Design review of the part built by this model. Coordinates are the model's own, in mm. Give positions to 0.01 mm unless a question says otherwise; leave off trailing zeros. Write each loop counter-clockwise with the first axis right and the second up, starting at its lowest first coordinate (ties: lowest second). Pieces come first, ordered by that corner, then holes. Notation, with made-up numbers: M 37,19 L 43,19 A23 ccw 43,36 Z; hole C -6,61 d1. An arc over 180 degrees is marked long. Use a Markdown table: item, result. Add a question column.
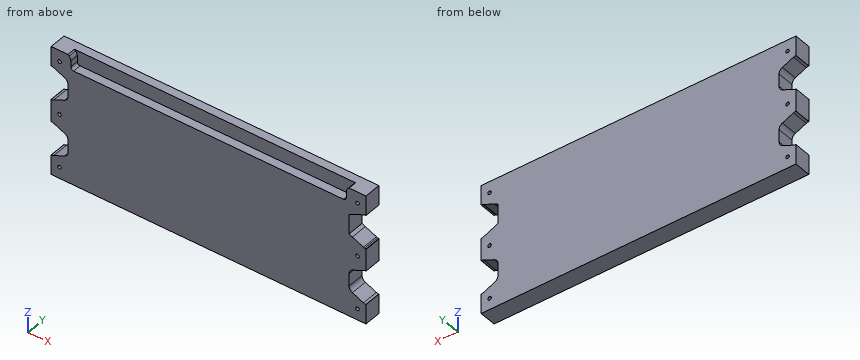
```python
from build123d import *

# Parameters (mm, degrees)
F0_R     = 1.984375
F1_DEPTH = 9.525
F2_DEPTH = 9.525
F3_SIZE  = 3.175
F4_R     = 6.35


# Not quite as in the source:
# - ends of sketch curves that miss each other by under 0.0002 mm in the source are joined


with BuildPart() as f1:
    # F0 (on Front) → F1 (new body)
    with BuildSketch(Plane.XZ):
        with BuildLine():
            ThreePointArc((106.6892375248, 39.5968594302), (108.9343015551, 40.5267953999), (109.8642375248, 42.7718594302))
            Line((109.8642375248, 42.7718594302), (109.8642375248, 55.4718594302))
            Line((109.8642375248, 55.4718594302), (-201.2857624752, 55.4718594302))
            Line((-201.2857624752, 55.4718594302), (-201.2857624752, 42.7718594302))
            ThreePointArc((-201.2857624752, 42.7718594302), (-200.3558265055, 40.5267953999), (-198.1107624752, 39.5968594302))
            Line((-198.1107624752, 39.5968594302), (106.6892375248, 39.5968594302))
        make_face()
        with BuildLine():
            Line((109.8642375248, 55.4718594302), (109.8642375248, 42.7718594302))
            ThreePointArc((109.8642375248, 42.7718594302), (108.9343015551, 40.5267953999), (106.6892375248, 39.5968594302))
            Line((106.6892375248, 39.5968594302), (-198.1107624752, 39.5968594302))
            ThreePointArc((-198.1107624752, 39.5968594302), (-200.3558265055, 40.5267953999), (-201.2857624752, 42.7718594302))
            Line((-201.2857624752, 42.7718594302), (-201.2857624752, 55.4718594302))
            Line((-201.2857624752, 55.4718594302), (-223.5107624752, 55.4718594302))
            Line((-223.5107624752, 55.4718594302), (-223.5107624752, 33.2468594302))
            Line((-223.5107624752, 33.2468594302), (-223.2986885503, 33.2468594302))
            ThreePointArc((-223.2986885503, 33.2468594302), (-221.9543922864, 33.1029344825), (-220.6710339026, 32.6776838569))
            Line((-220.6710339026, 32.6776838569), (-208.1831078275, 27.0013383101))
            ThreePointArc((-208.1831078275, 27.0013383101), (-205.471843717, 24.6583106333), (-204.4607624752, 21.2205138834))
            Line((-204.4607624752, 21.2205138834), (-204.4607624752, 7.1731958926))
            ThreePointArc((-204.4607624752, 7.1731958926), (-205.4718446589, 3.7353976799), (-208.1831109951, 1.392370026))
            Line((-208.1831109951, 1.392370026), (-220.6710352489, -4.2839664363))
            ThreePointArc((-220.6710352489, -4.2839664363), (-221.9543921654, -4.7092159904), (-223.298686729, -4.8531405698))
            Line((-223.298686729, -4.8531405698), (-223.5107370752, -4.8531405698))
            Line((-223.5107370752, -4.8531405698), (-223.5107624752, -30.2531405698))
            Line((-223.5107624752, -30.2531405698), (-223.298686729, -30.2531405698))
            ThreePointArc((-223.298686729, -30.2531405698), (-221.9543921654, -30.3970651492), (-220.6710352489, -30.8223147033))
            Line((-220.6710352489, -30.8223147033), (-208.1831109951, -36.4986511657))
            ThreePointArc((-208.1831109951, -36.4986511657), (-205.4718446589, -38.8416788196), (-204.4607624752, -42.2794770322))
            Line((-204.4607624752, -42.2794770322), (-204.4607624752, -56.326795023))
            ThreePointArc((-204.4607624752, -56.326795023), (-205.471843717, -59.7645917729), (-208.1831078275, -62.1076194497))
            Line((-208.1831078275, -62.1076194497), (-220.6710339026, -67.7839649965))
            ThreePointArc((-220.6710339026, -67.7839649965), (-221.9543922864, -68.2092156221), (-223.2986885503, -68.3531405698))
            Line((-223.2986885503, -68.3531405698), (-223.5107370752, -68.3531405698))
            Line((-223.5107370752, -68.3531405698), (-223.5107624752, -90.5781405698))
            Line((-223.5107624752, -90.5781405698), (132.0892375248, -90.5781405698))
            Line((132.0892375248, -90.5781405698), (132.0892375248, -68.3531405698))
            Line((132.0892375248, -68.3531405698), (131.8771635999, -68.3531405698))
            ThreePointArc((131.8771635999, -68.3531405698), (130.532867336, -68.2092156221), (129.2495089522, -67.7839649965))
            Line((129.2495089522, -67.7839649965), (116.7615828771, -62.1076194497))
            ThreePointArc((116.7615828771, -62.1076194497), (114.0503187666, -59.7645917729), (113.0392375248, -56.326795023))
            Line((113.0392375248, -56.326795023), (113.0392375248, -42.2794770322))
            ThreePointArc((113.0392375248, -42.2794770322), (114.0503197085, -38.8416788196), (116.7615860447, -36.4986511657))
            Line((116.7615860447, -36.4986511657), (129.2495102985, -30.8223147033))
            ThreePointArc((129.2495102985, -30.8223147033), (130.5328672149, -30.3970651492), (131.8771617786, -30.2531405698))
            Line((131.8771617786, -30.2531405698), (132.0892121248, -30.2531405698))
            Line((132.0892121248, -30.2531405698), (132.0892375248, -5.5747531892))
            Line((132.0892375248, -5.5747531892), (130.5016917914, -4.8531405698))
            Line((130.5016917914, -4.8531405698), (129.2495102985, -4.2839664363))
            Line((129.2495102985, -4.2839664363), (116.7615860447, 1.392370026))
            Line((116.7615860447, 1.392370026), (113.0392375248, 3.0843487889))
            Line((113.0392375248, 3.0843487889), (113.0392375248, 7.1731958926))
            Line((113.0392375248, 7.1731958926), (113.0392375248, 21.2205138834))
            Line((113.0392375248, 21.2205138834), (113.0392375248, 25.3093700715))
            Line((113.0392375248, 25.3093700715), (116.7615794549, 27.001345839))
            Line((116.7615794549, 27.001345839), (129.2495086403, 32.677684543))
            Line((129.2495086403, 32.677684543), (130.5016917914, 33.2468594302))
            Line((130.5016917914, 33.2468594302), (132.0892375248, 33.9684720496))
            Line((132.0892375248, 33.9684720496), (132.0892375248, 55.4718594302))
            Line((132.0892375248, 55.4718594302), (109.8642375248, 55.4718594302))
        make_face()
        with Locations((-213.9857624752, -77.8781405698)):
            Circle(F0_R, mode=Mode.SUBTRACT)
        with Locations((122.5642375248, -77.8781405698)):
            Circle(F0_R, mode=Mode.SUBTRACT)
        with Locations((-213.9857624752, -17.5531402737)):
            Circle(F0_R, mode=Mode.SUBTRACT)
        with Locations((-213.9857624752, 42.7718594302)):
            Circle(F0_R, mode=Mode.SUBTRACT)
        with Locations((122.5642375248, -17.5531402737)):
            Circle(F0_R, mode=Mode.SUBTRACT)
        with Locations((122.5642375248, 42.7718594302)):
            Circle(F0_R, mode=Mode.SUBTRACT)
        Polygon((132.0892375248, 33.2468594302), (132.0892375248, 33.9684720496), (130.5016917914, 33.2468594302), (131.8771635999, 33.2468594302), align=None)
        Polygon((132.0892375248, -5.5747531892), (132.0892375248, -4.8531405698), (131.8771617786, -4.8531405698), (130.5016917914, -4.8531405698), align=None)
    extrude(amount=-F1_DEPTH)

    # F0 (on Front) → F2 (join)
    with BuildSketch(Plane.XZ):
        with BuildLine():
            Line((109.8642375248, 55.4718594302), (109.8642375248, 42.7718594302))
            ThreePointArc((109.8642375248, 42.7718594302), (108.9343015551, 40.5267953999), (106.6892375248, 39.5968594302))
            Line((106.6892375248, 39.5968594302), (-198.1107624752, 39.5968594302))
            ThreePointArc((-198.1107624752, 39.5968594302), (-200.3558265055, 40.5267953999), (-201.2857624752, 42.7718594302))
            Line((-201.2857624752, 42.7718594302), (-201.2857624752, 55.4718594302))
            Line((-201.2857624752, 55.4718594302), (-223.5107624752, 55.4718594302))
            Line((-223.5107624752, 55.4718594302), (-223.5107624752, 33.2468594302))
            Line((-223.5107624752, 33.2468594302), (-223.2986885503, 33.2468594302))
            ThreePointArc((-223.2986885503, 33.2468594302), (-221.9543922864, 33.1029344825), (-220.6710339026, 32.6776838569))
            Line((-220.6710339026, 32.6776838569), (-208.1831078275, 27.0013383101))
            ThreePointArc((-208.1831078275, 27.0013383101), (-205.471843717, 24.6583106333), (-204.4607624752, 21.2205138834))
            Line((-204.4607624752, 21.2205138834), (-204.4607624752, 7.1731958926))
            ThreePointArc((-204.4607624752, 7.1731958926), (-205.4718446589, 3.7353976799), (-208.1831109951, 1.392370026))
            Line((-208.1831109951, 1.392370026), (-220.6710352489, -4.2839664363))
            ThreePointArc((-220.6710352489, -4.2839664363), (-221.9543921654, -4.7092159904), (-223.298686729, -4.8531405698))
            Line((-223.298686729, -4.8531405698), (-223.5107370752, -4.8531405698))
            Line((-223.5107370752, -4.8531405698), (-223.5107624752, -30.2531405698))
            Line((-223.5107624752, -30.2531405698), (-223.298686729, -30.2531405698))
            ThreePointArc((-223.298686729, -30.2531405698), (-221.9543921654, -30.3970651492), (-220.6710352489, -30.8223147033))
            Line((-220.6710352489, -30.8223147033), (-208.1831109951, -36.4986511657))
            ThreePointArc((-208.1831109951, -36.4986511657), (-205.4718446589, -38.8416788196), (-204.4607624752, -42.2794770322))
            Line((-204.4607624752, -42.2794770322), (-204.4607624752, -56.326795023))
            ThreePointArc((-204.4607624752, -56.326795023), (-205.471843717, -59.7645917729), (-208.1831078275, -62.1076194497))
            Line((-208.1831078275, -62.1076194497), (-220.6710339026, -67.7839649965))
            ThreePointArc((-220.6710339026, -67.7839649965), (-221.9543922864, -68.2092156221), (-223.2986885503, -68.3531405698))
            Line((-223.2986885503, -68.3531405698), (-223.5107370752, -68.3531405698))
            Line((-223.5107370752, -68.3531405698), (-223.5107624752, -90.5781405698))
            Line((-223.5107624752, -90.5781405698), (132.0892375248, -90.5781405698))
            Line((132.0892375248, -90.5781405698), (132.0892375248, -68.3531405698))
            Line((132.0892375248, -68.3531405698), (131.8771635999, -68.3531405698))
            ThreePointArc((131.8771635999, -68.3531405698), (130.532867336, -68.2092156221), (129.2495089522, -67.7839649965))
            Line((129.2495089522, -67.7839649965), (116.7615828771, -62.1076194497))
            ThreePointArc((116.7615828771, -62.1076194497), (114.0503187666, -59.7645917729), (113.0392375248, -56.326795023))
            Line((113.0392375248, -56.326795023), (113.0392375248, -42.2794770322))
            ThreePointArc((113.0392375248, -42.2794770322), (114.0503197085, -38.8416788196), (116.7615860447, -36.4986511657))
            Line((116.7615860447, -36.4986511657), (129.2495102985, -30.8223147033))
            ThreePointArc((129.2495102985, -30.8223147033), (130.5328672149, -30.3970651492), (131.8771617786, -30.2531405698))
            Line((131.8771617786, -30.2531405698), (132.0892121248, -30.2531405698))
            Line((132.0892121248, -30.2531405698), (132.0892375248, -5.5747531892))
            Line((132.0892375248, -5.5747531892), (130.5016917914, -4.8531405698))
            Line((130.5016917914, -4.8531405698), (129.2495102985, -4.2839664363))
            Line((129.2495102985, -4.2839664363), (116.7615860447, 1.392370026))
            Line((116.7615860447, 1.392370026), (113.0392375248, 3.0843487889))
            Line((113.0392375248, 3.0843487889), (113.0392375248, 7.1731958926))
            Line((113.0392375248, 7.1731958926), (113.0392375248, 21.2205138834))
            Line((113.0392375248, 21.2205138834), (113.0392375248, 25.3093700715))
            Line((113.0392375248, 25.3093700715), (116.7615794549, 27.001345839))
            Line((116.7615794549, 27.001345839), (129.2495086403, 32.677684543))
            Line((129.2495086403, 32.677684543), (130.5016917914, 33.2468594302))
            Line((130.5016917914, 33.2468594302), (132.0892375248, 33.9684720496))
            Line((132.0892375248, 33.9684720496), (132.0892375248, 55.4718594302))
            Line((132.0892375248, 55.4718594302), (109.8642375248, 55.4718594302))
        make_face()
        with Locations((-213.9857624752, -77.8781405698)):
            Circle(F0_R, mode=Mode.SUBTRACT)
        with Locations((122.5642375248, -77.8781405698)):
            Circle(F0_R, mode=Mode.SUBTRACT)
        with Locations((-213.9857624752, -17.5531402737)):
            Circle(F0_R, mode=Mode.SUBTRACT)
        with Locations((-213.9857624752, 42.7718594302)):
            Circle(F0_R, mode=Mode.SUBTRACT)
        with Locations((122.5642375248, -17.5531402737)):
            Circle(F0_R, mode=Mode.SUBTRACT)
        with Locations((122.5642375248, 42.7718594302)):
            Circle(F0_R, mode=Mode.SUBTRACT)
        Polygon((132.0892375248, 33.2468594302), (132.0892375248, 33.9684720496), (130.5016917914, 33.2468594302), (131.8771635999, 33.2468594302), align=None)
        Polygon((132.0892375248, -5.5747531892), (132.0892375248, -4.8531405698), (131.8771617786, -4.8531405698), (130.5016917914, -4.8531405698), align=None)
    extrude(amount=F2_DEPTH)

    # F3
    f3_edges = [f1.edges().sort_by_distance(p)[0] for p in [
        (-201.285762, -4.7625, 55.471859),
        (109.864238, -4.7625, 55.471859),
    ]]
    chamfer(f3_edges, length=F3_SIZE)

    # F4
    f4_edges = [f1.edges().sort_by_distance(p)[0] for p in [
        (109.864238, -4.7625, 52.296859),
        (-201.285762, -4.7625, 52.296859),
    ]]
    fillet(f4_edges, radius=F4_R)


solid = f1.part
```
(1) For pin 1 (3 mm diameter, centred on x = -213.99, z = 42.77, fed in from -Y); pin 2 (3 mm diameter, centred on x = -71.5, y = -5, fed in from +Z); pin 3 (2 mm diameter, centred on y = 7.5, z = -48.5, fed in from -X); pin 4 (6.5 mm diameter, centred on x = -213.99, z = -17.55, fed in from +Y) (3 decimals), all flat-tipped, find the tip position at first contact; note any pin that passes through.
(2) Add section B-B on y = 6.5. Give the number of separate pieces and of enclosed holes in the cut face, then the cut area to 3 significant figures.
(3) Add section A-A on x = -10. Give the boundary of the cut face in (y, z) (3 decimals), then the cut area to 3 significant figures.
(4) Wall thickness on L1, parallel to X at y = -3.5, z = 46; L2, parallel to Z at x = -85, y = -3.5; L3, parallel to X at y = 0.5, z = -42: over which ranges is each line inside the solid? List them lowest first.
From the geometry:
| question | item | result |
|---|---|---|
| 1 | pin 1 | passes through |
| 1 | pin 2 | stops at z = 39.6 |
| 1 | pin 3 | stops at x = -204.46 |
| 1 | pin 4 | stops at y = 9.525 |
| 2 | separate pieces | 1 |
| 2 | enclosed holes | 6 |
| 2 | area | 49,500 mm^2 |
| 3 | outline | M -9.525,-90.578 L 9.525,-90.578 L 9.525,55.472 L 0,55.472 L 0,39.597 L -9.525,39.597 Z |
| 3 | area | 2,630 mm^2 |
| 4 | L1 | x = -223.51 to -201.29, 109.86 to 132.09 |
| 4 | L2 | z = -90.58 to 39.6 |
| 4 | L3 | x = -204.47 to 113.05 |
